The model under review builds one solid part; all positions refer to its coordinate system, in mm. Face numbers are marked on the shaded views. Coordinates: 2 decimals unless noted, no trailing zeros. Order: outer loops, then holes, each group sorted by start corner. A loop starts at its lowest first (then second) coordinate and runs counter-clockwise, first axis right, second up. Notation, with made-up numbers: (1, 79) -> (9, 79) arc R23 cw to (9, 105) -> close; hole circle Ø2 at (4.25, 79.5). An arc over 180 degrees is marked (long way). Use one line per item in the form item = value.
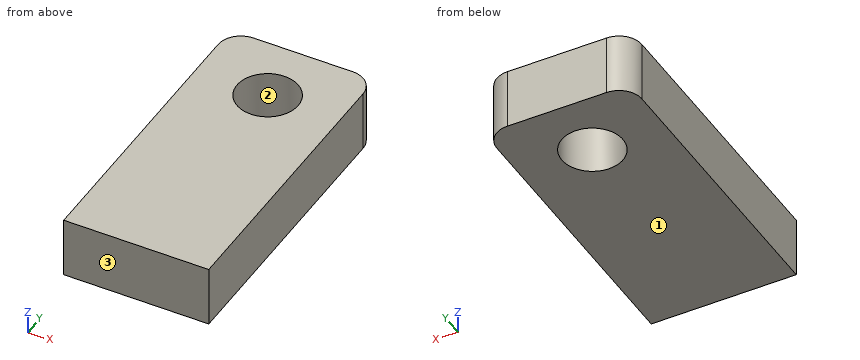
Autodesk Inventor part; units mm, degrees
ref_plane "YZ Plane" through (0, 0, 0) normal (1, 0, 0) x (0, 1, 0)
ref_plane "XZ Plane" through (0, 0, 0) normal (0, 1, 0) x (-1, 0, 0)
ref_plane "XY Plane" through (0, 0, 0) normal (0, 0, 1) x (1, 0, 0)
sketch "Sketch2" plane through (0, 0, 0) normal (0, 0, 1) x (1, 0, 0)
  line L0 (-9.5, -20) -> (9.5, -20)
  line L1 (9.5, -20) -> (9.5, 17)
  line L2 (6.5, 20) -> (-6.5, 20)
  line L3 (-9.5, 17) -> (-9.5, -20)
  line L4 (-9.5, -20) -> (9.5, 20) construction
  line L5 (9.5, -20) -> (-9.5, 20) construction
  arc A0 (-6.5, 20) -> (-9.5, 17) centre (-6.5, 17) ccw
  arc A1 (9.5, 17) -> (6.5, 20) centre (6.5, 17) ccw
  line L6 (0, 20) -> (0, 11.5)
  circle A2 centre (0, 11.5) radius 4
  point P0 (0, 0)
  dimension "d7" = 19
  dimension "d8" = 40
  dimension "d9" = 3
  dimension "d10" = 8.5
  dimension "d11" = 8
extrude "Extrusion2" add sketch "Sketch2" along normal blind 8
thread "Thread1"
properties part number "Kengyel2"
Item 1: To check wall thickness, follow L1, parallel to Y at x = 0, z = 2.25; L2, parallel to Y at x = 1.5, z = 3.5; L3, parallel to X at y = 18.5, z = 1. State the ranges of each line that lie inside material, in increasing order. Write a range as from..to.
Results found:
L1 = -20..7.5, 15.5..20
L2 = -20..7.79, 15.21..20
L3 = -9.1..9.1
Item 2: Draft analysis for pull direction Y (two halves, no side actions). For the marked faces 1, 2 and 3, state which applies: released by +Y, released by -Y, zero draft, split by the parting line, or undercut.
Results found:
face_1 = zero draft
face_2 = undercut
face_3 = released by -Y
Item 3: We need section A-A (y = 11.5). Write out the cut boundary in (x, z).
Results found:
outline = (-9.5, 0) -> (-4, 0) -> (-4, 8) -> (-9.5, 8) -> close; (4, 0) -> (9.5, 0) -> (9.5, 8) -> (4, 8) -> close
Item 4: We need section B-B (z = 5.75). Write out the cut boundary in (x, y), plus the area to 3 significant figures.
Results found:
outline = (-9.5, -20) -> (9.5, -20) -> (9.5, 17) arc R3 ccw to (6.5, 20) -> (-6.5, 20) arc R3 ccw to (-9.5, 17) -> close; hole circle Ø8 at (0, 11.5)
area = 706 mm²
Item 5: We need section C-C (x = 0). Write out the cut boundary in (y, z).
Results found:
outline = (-20, 0) -> (7.5, 0) -> (7.5, 8) -> (-20, 8) -> close; (15.5, 0) -> (20, 0) -> (20, 8) -> (15.5, 8) -> close
